```python
from build123d import *

# Parameters (mm, degrees)
SKETCH1_R                = 40
SKETCH1_R_2              = 35
BOSS_EXTRUDE1_DEPTH      = 2
BOSS_EXTRUDE2_DEPTH      = 2
SKETCH3_R                = 3
CUT_EXTRUDE1_DEPTH       = 2
FILLET1_R                = 5
CIRPATTERN1_COUNT        = 3
FILLET1_OF_CIRPATTERN1_R = 5
SKETCH4_R                = 3
BOSS_EXTRUDE3_DEPTH      = 2
FILLET2_R                = 4
CIRPATTERN2_COUNT        = 3
FILLET2_OF_CIRPATTERN2_R = 4


with BuildPart() as part:
    # Sketch1 → Boss-Extrude1 (new body)
    with BuildSketch(Plane.XY):
        Circle(SKETCH1_R)
        Circle(SKETCH1_R_2, mode=Mode.SUBTRACT)
    extrude(amount=BOSS_EXTRUDE1_DEPTH)

    # Sketch2 → Boss-Extrude2 (add)
    with BuildSketch(Plane(origin=(0, 0, 0), x_dir=(-1, 0, 0), z_dir=(0, 0, -1))):
        with BuildLine():
            Line((-29, -5), (-34.641016151, -5))
            Line((-34.641016151, -5), (-37, -5))
            Line((-37, -5), (-37, 5))
            Line((-37, 5), (-34.641016151, 5))
            Line((-34.641016151, 5), (-29, 5))
            ThreePointArc((-29, 5), (-24, 0), (-29, -5))
        make_face()
        with BuildLine():
            Line((-34, -3), (-29, -3))
            ThreePointArc((-29, -3), (-26, 0), (-29, 3))
            Line((-29, 3), (-34, 3))
            ThreePointArc((-34, 3), (-37, 0), (-34, -3))
        make_face(mode=Mode.SUBTRACT)
    boss_extrude2 = extrude(amount=-BOSS_EXTRUDE2_DEPTH)

    # Sketch3 → Cut-Extrude1 (cut)
    with BuildSketch(Plane(origin=(0, 0, 0), x_dir=(-1, 0, 0), z_dir=(0, 0, -1))):
        with Locations((-34, 0)):
            Circle(SKETCH3_R)
    cut_extrude1 = extrude(amount=-CUT_EXTRUDE1_DEPTH, mode=Mode.SUBTRACT)

    # Fillet1
    fillet1_edges = [part.edges().sort_by_distance(p)[0] for p in [
        (34.641016151, -5, 1),
        (34.641016151, 5, 1),
    ]]
    fillet(fillet1_edges, radius=FILLET1_R)

    # CirPattern1: Boss-Extrude2, Cut-Extrude1 ×3 about axis
    cirpattern1_axis = Axis((0, 0, 0), (0, 0, 1))
    for i in range(1, CIRPATTERN1_COUNT):
        add(boss_extrude2.rotate(cirpattern1_axis, i * 360 / CIRPATTERN1_COUNT))
        add(cut_extrude1.rotate(cirpattern1_axis, i * 360 / CIRPATTERN1_COUNT), mode=Mode.SUBTRACT)

    # Fillet1 of CirPattern1
    fillet1_of_cirpattern1_edges = [part.edges().sort_by_distance(p)[0] for p in [
        (-12.990381057, 32.5, 1),
        (-21.650635095, 27.5, 1),
        (-21.650635095, -27.5, 1),
        (-12.990381057, -32.5, 1),
    ]]
    fillet(fillet1_of_cirpattern1_edges, radius=FILLET1_OF_CIRPATTERN1_R)

    # Sketch4 → Boss-Extrude3 (add)
    with BuildSketch(Plane(origin=(0, 0, 0), x_dir=(-1, 0, 0), z_dir=(0, 0, -1))):
        with BuildLine():
            Line((-15.513007814, 36.869317712), (-18.669872981, 42.337168574))
            ThreePointArc((-18.669872981, 42.337168574), (-25.5, 44.167295593), (-27.330127019, 37.337168574))
            Line((-27.330127019, 37.337168574), (-24.173261852, 31.869317712))
            Line((-24.173261852, 31.869317712), (-15.513007814, 36.869317712))
        make_face()
        with Locations((-23, 39.837168574)):
            Circle(SKETCH4_R, mode=Mode.SUBTRACT)
    boss_extrude3 = extrude(amount=-BOSS_EXTRUDE3_DEPTH)

    # Fillet2
    fillet2_edges = [part.edges().sort_by_distance(p)[0] for p in [
        (15.513007814, 36.869317712, 1),
        (24.173261852, 31.869317712, 1),
    ]]
    fillet(fillet2_edges, radius=FILLET2_R)

    # CirPattern2: Boss-Extrude3 ×3 about axis
    cirpattern2_axis = Axis((0, 0, 0), (0, 0, 1))
    for i in range(1, CIRPATTERN2_COUNT):
        add(boss_extrude3.rotate(cirpattern2_axis, i * 360 / CIRPATTERN2_COUNT))

    # Fillet2 of CirPattern2
    fillet2_of_cirpattern2_edges = [part.edges().sort_by_distance(p)[0] for p in [
        (-39.686269666, -5, 1),
        (-39.686269666, 5, 1),
        (24.173261852, -31.869317712, 1),
        (15.513007814, -36.869317712, 1),
    ]]
    fillet(fillet2_of_cirpattern2_edges, radius=FILLET2_OF_CIRPATTERN2_R)


solid = part.part
```
Geometry: final body of the model. Coordinates: model frame, mm. A direction names the side the tool comes from. Round coordinates to 2 decimals unless told otherwise and drop trailing zeros. Write each loop counter-clockwise with the first axis right and the second up, starting at its lowest first coordinate (ties: lowest second). Pieces come first, ordered by that corner, then holes.
Item 1: Pin query (flat end, axial travel): P1, Ø1, axis at y = -32, z = 1.5, coming from the +X side; P2, Ø1, axis at y = -31, z = 1.5, coming from the +X side; P3, Ø0.6, axis at x = -45, z = 1, coming from the +Y side. Return the tip coordinate at first contact, or that it passes through.
Item 2: Section query B-B (y = 1). Return loops of the section in (x, z), plus the area to 3 significant figures.
Item 3: Section query D-D (z = 1.25). Give the number of separate pieces and of enclosed holes in the cut face, plus the area to 3 significant figures.
Item 4: Section query C-C (x = -15.5). Return loops of the section in (y, z).
Item 5: Section query A-A (x = -32). Return loops of the section in (y, z), plus the area to 3 significant figures.
Item 6: Set-up query: faces 1 (the face through (17.2, -30.48, 0.99)), 2 (the face through (40, 0, 1)). Return all of +Z, -Z, +X, -X, +Y, -Y with unobstructed straight access to the full face (end or side cutting, diameter ignored); none if empty.
Item 7: Material intervals for L1, parallel to X at y = 21.5, z = 1; L2, parallel to Y at x = 23, z = 1.3; L3, parallel to X at y = 0.5, z = 1.7, sorted ascending.
Item 8: Mould query, pull axis Y, two halves, no side actions, for faces 3 (the face through (-51, 0, 1)), 4 (the face through (23.39, 42.81, 0.99)), 5 (the face through (17.927, 41.051, 0.986)). Classes: +Y half, -Y half, draft (parallel to the pull), parting line (faces both ways), or undercut.
Completed:
1. P1: stops at x = 25.55
1. P2: stops at x = 26.06
1. P3: stops at y = 5
2. outline: (-50.9, 0) - (-48.83, 0) - (-48.83, 2) - (-50.9, 2) - close; (-43.17, 0) - (-34.99, 0) - (-34.99, 2) - (-43.17, 2) - close; (24.1, 0) - (26.17, 0) - (26.17, 2) - (24.1, 2) - close; (36.83, 0) - (39.99, 0) - (39.99, 2) - (36.83, 2) - close
2. area: 31.0 mm2
3. separate pieces: 1
3. enclosed holes: 7
3. area: 1,590 mm2
4. outline: (-36.87, 0) - (-32.04, 0) - (-32.04, 2) - (-36.87, 2) - close; (-22.29, 0) - (-20.22, 0) - (-20.22, 2) - (-22.29, 2) - close; (20.22, 0) - (22.29, 0) - (22.29, 2) - (20.22, 2) - close; (32.04, 0) - (36.87, 0) - (36.87, 2) - (32.04, 2) - close
5. outline: (-24, 0) - (-14.18, 0) - (-14.18, 2) - (-24, 2) - close; (14.18, 0) - (24, 0) - (24, 2) - (14.18, 2) - close
5. area: 39.3 mm2
6. face 1: +Z, -Z
6. face 2: +Z, -Z, +X
7. L1: x = -33.73 to -27.62, -17.95 to -11.05, 27.62 to 33.73
7. L2: y = -44.84 to -42.84, -36.84 to -26.38, 26.38 to 36.84, 42.84 to 44.84
7. L3: x = -50.97 to -48.96, -43.04 to -35, 24.03 to 26.04, 36.96 to 40
8. face 3: parting line
8. face 4: undercut
8. face 5: +Y half
